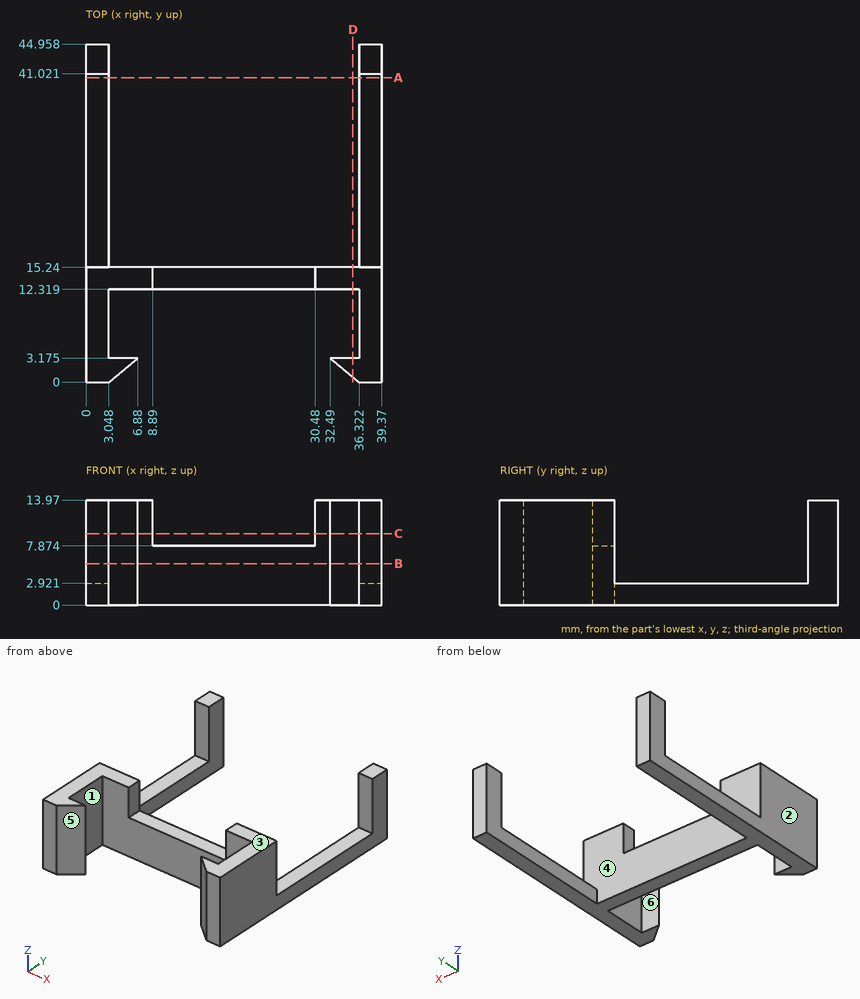
Study the drawing (mm; zero at the part's minimum x, y, z) and answer. A direction names the side the tool comes from. Round coordinates to 2 decimals unless told otherwise and drop trailing zeros. Order: outer loops, then holes, each group sorted by start corner. A loop starts at its lowest first (then second) coordinate and runs counter-clockwise, first axis right, second up. Notation, with made-up numbers: (0.5, 13.25) -> (27.5, 13.25) arc R17 ccw to (27.5, 18.25) -> close; hole circle Ø8 at (83.5, 87). An arc over 180 degrees is marked (long way). Answer as CSV lines item,"result". Start each with the question number.
(1) The part is cut by section B-B (z = 5.5). Determine the outline of the cut face in (x, y) (1 decimal).
(2) A tool of negligible diameter and unlimited length cuts with its end or side. For the marked faces 4, 5 and 6, from which of +Z, -Z, +X, -X, +Y, -Y can it reach the whole face along a straight path? Write none if from no direction.
(3) Flat-ended cylindrical pins translate along their axes: pin 1 Ø4 at (x, z) = (24, 10.5) entering from -Y (1 decimal); pin 2 Ø2.5 at (x, y) = (37, 28.5) entering from +Z; pin 3 Ø4 at (x, z) = (34, 8) entering from +Y; pin 4 Ø2 at (x, z) = (30, 11) entering from -Y. Find the tip coordinate at first contact, or state that the pin passes through.
(4) The part is cut by section D-D (x = 35.5). Determine the outline of the cut face in (y, z) (1 decimal).
(5) For a pull along X with two mould halves and no side action, classify the marked faces 1, 2 and 3 as +X half, -X half, draft (parallel to the pull), parting line (faces both ways), or undercut.
(6) The part is cut by section A-A (y = 40.5). Determine the outline of the cut face in (x, z).
(7) Find the intervals of material crossed by probe 1 along X at (y, z) = (34.5, 1.25); probe 2 along Y at (x, z) = (37, 4); probe 3 along Y at (x, z) = (16, 7.75), in increasing order. Write a range as from..to.
(8) The part is cut by section C-C (z = 9.5). Determine the outline of the cut face in (x, y) (1 decimal).
Evaluation:
1,outline,"(0, 0) -> (3, 0) -> (6.9, 3.2) -> (3, 3.2) -> (3, 12.3) -> (36.3, 12.3) -> (36.3, 3.2) -> (32.5, 3.2) -> (36.3, 0) -> (39.4, 0) -> (39.4, 15.2) -> (0, 15.2) -> close; (0, 41) -> (3, 41) -> (3, 45) -> (0, 45) -> close; (36.3, 41) -> (39.4, 41) -> (39.4, 45) -> (36.3, 45) -> close"
2,face 4,"+Z"
2,face 5,"+Z, -Z, -Y"
2,face 6,"+Z, -Z"
3,pin 1,"through"
3,pin 2,"z = 2.92"
3,pin 3,"y = 15.24"
3,pin 4,"y = 12.32"
4,outline,"(0.7, 0) -> (3.2, 0) -> (3.2, 14) -> (0.7, 14) -> close; (12.3, 0) -> (15.2, 0) -> (15.2, 14) -> (12.3, 14) -> close"
5,face 1,"undercut"
5,face 2,"-X half"
5,face 3,"draft"
6,outline,"(0, 0) -> (3.05, 0) -> (3.05, 2.92) -> (0, 2.92) -> close; (36.32, 0) -> (39.37, 0) -> (39.37, 2.92) -> (36.32, 2.92) -> close"
7,probe 1,"0..3.05, 36.32..39.37"
7,probe 2,"0..15.24, 41.02..44.96"
7,probe 3,"12.32..15.24"
8,outline,"(0, 0) -> (3, 0) -> (6.9, 3.2) -> (3, 3.2) -> (3, 12.3) -> (8.9, 12.3) -> (8.9, 15.2) -> (0, 15.2) -> close; (0, 41) -> (3, 41) -> (3, 45) -> (0, 45) -> close; (30.5, 12.3) -> (36.3, 12.3) -> (36.3, 3.2) -> (32.5, 3.2) -> (36.3, 0) -> (39.4, 0) -> (39.4, 15.2) -> (30.5, 15.2) -> close; (36.3, 41) -> (39.4, 41) -> (39.4, 45) -> (36.3, 45) -> close"
